Build history of the part. All positions in model axes, mm. Face numbers are marked on the shaded views. A direction names the side the tool comes from. Coordinates: 2 decimals unless noted, no trailing zeros. Loops run counter-clockwise (first coordinate to the right, second up) from the corner with the lowest first, then second, coordinate; pieces in that order, holes last.
Item 1: Cut at C-C (y = -8.5). List the corners of the cut face in (x, z).
Item 2: Drill centre lines: line 1 along X through (y, z) = (4.5, -10); line 2 along Y through (x, z) = (2.5, -13.5); line 3 along Z through (x, y) = (0, 6). Where is each one in solid material? Low to high.
Item 3: 3-axis set-ups, long thin cutter, end or side, ignore diameter. For the marked faces 1, 2, 3 and 4: which of +Z, -Z, +X, -X, +Y, -Y reach the whole face in a straight line?
Item 4: Cut at A-A (z = -8). List the corners of the cut face in (x, y).
Item 5: Cut at D-D (x = -9). List the corners of the cut face in (y, z).
Item 6: Cut at B-B (x = 0). List the corners of the cut face in (y, z), and give its area (3 significant figures).
Item 7: Flat gauge pins, fed straight in: pin 1 (6.5 mm diameter, centred on x = 0, z = -10, fed in from +Y); pin 2 (2.5 mm diameter, centred on x = -1.5, y = 1, fed in from -Z); pin 3 (5 mm diameter, centred on y = 4, z = -5.5, fed in from +X); pin 4 (6 mm diameter, centred on y = -14, z = -7.5, fed in from +X). Where does each tip first touch, or does it go through?
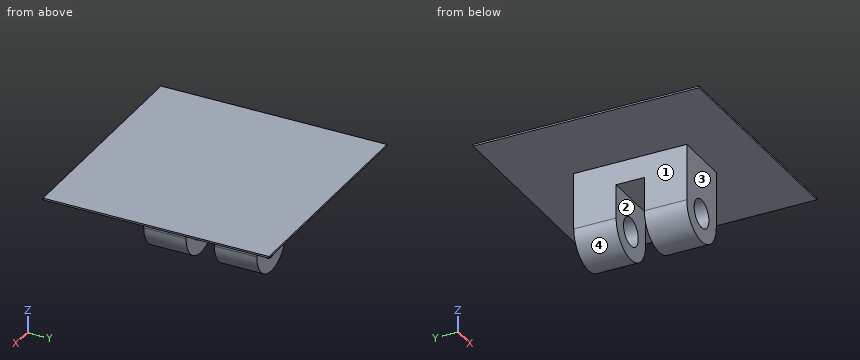
from build123d import *

# Parameters (mm, degrees)
CROQUIS1_W                   = 40
CROQUIS1_H                   = 40
SALIENTE_EXTRUIR1_DEPTH      = 0.3
SALIENTE_EXTRUIR2_DEPTH      = 10
SALIENTE_EXTRUIR2_DEPTH_BACK = 10
CROQUIS2_R                   = 2.5
CORTAR_EXTRUIR1_DEPTH        = 2.5
CORTAR_EXTRUIR1_DEPTH_BACK   = 2.5
CROQUIS3_W                   = 14.056155144
CROQUIS3_H                   = 12


with BuildPart() as part:
    # Croquis1 → Saliente-Extruir1 (new body)
    with BuildSketch(Plane.XY):
        Rectangle(CROQUIS1_W, CROQUIS1_H)
    extrude(amount=SALIENTE_EXTRUIR1_DEPTH)

    # Croquis2 → Saliente-Extruir2 (add, two sides: drawn at the far end of the back side and taken through both)
    with BuildSketch(Plane(origin=(0, 0, 0), x_dir=(1, 0, 0), z_dir=(0, 1, 0)).offset(-SALIENTE_EXTRUIR2_DEPTH_BACK)):
        with BuildLine():
            Line((-5, 10), (-5, 0))
            Line((-5, 0), (5, 0))
            Line((5, 0), (5, 10))
            ThreePointArc((5, 10), (0, 15), (-5, 10))
        make_face()
        with Locations(Location((0, 10, 0), (0, 0, 270))):
            Circle(CROQUIS2_R, mode=Mode.SUBTRACT)
    extrude(amount=SALIENTE_EXTRUIR2_DEPTH + SALIENTE_EXTRUIR2_DEPTH_BACK)

    # Croquis3 → Cortar-Extruir1 (cut, two sides: drawn at the far end of the back side and taken through both)
    with BuildSketch(Plane(origin=(0, 0, 0), x_dir=(1, 0, 0), z_dir=(0, 1, 0)).offset(-CORTAR_EXTRUIR1_DEPTH_BACK)):
        with Locations((0, 10)):
            Rectangle(CROQUIS3_W, CROQUIS3_H)
    extrude(amount=CORTAR_EXTRUIR1_DEPTH + CORTAR_EXTRUIR1_DEPTH_BACK, mode=Mode.SUBTRACT)


solid = part.part
Filled sheet:
1. outline: (-20, 0) - (-5, 0) - (-5, -10) arc R5 ccw to (5, -10) - (5, 0) - (20, 0) - (20, 0.3) - (-20, 0.3) - close; hole circle Ø5 at (0, -10)
2. line 1: x = -5 to -2.5, 2.5 to 5
2. line 2: y = -10 to -2.5, 2.5 to 10
2. line 3: z = -15 to -12.5, -7.5 to 0.3
3. face 1: -Z, -X, +Y, -Y
3. face 2: -Z, +X, -X
3. face 3: -Z, +X, -X, -Y
3. face 4: -Z, +Y, -Y
4. outline: (-5, -10) - (-1.5, -10) - (-1.5, -2.5) - (-5, -2.5) - close; (-5, 2.5) - (-1.5, 2.5) - (-1.5, 10) - (-5, 10) - close; (1.5, -10) - (5, -10) - (5, -2.5) - (1.5, -2.5) - close; (1.5, 2.5) - (5, 2.5) - (5, 10) - (1.5, 10) - close
5. outline: (-20, 0) - (20, 0) - (20, 0.3) - (-20, 0.3) - close
6. outline: (-20, 0) - (-10, 0) - (-10, -7.5) - (-2.5, -7.5) - (-2.5, -4) - (2.5, -4) - (2.5, -7.5) - (10, -7.5) - (10, 0) - (20, 0) - (20, 0.3) - (-20, 0.3) - close; (-10, -15) - (-2.5, -15) - (-2.5, -12.5) - (-10, -12.5) - close; (2.5, -15) - (10, -15) - (10, -12.5) - (2.5, -12.5) - close
6. area: 182 mm2
7. pin 1: stops at y = 10
7. pin 2: stops at z = -4
7. pin 3: stops at x = 5
7. pin 4: passes through
